from build123d import *

# Parameters (mm, degrees)
SKETCH1_R           = 1.96
BOSS_EXTRUDE1_DEPTH = 20
SKETCH2_R           = 3.45
BOSS_EXTRUDE2_DEPTH = 4
CUT_EXTRUDE1_DEPTH  = 2.7
FILLET1_R           = 0.2


with BuildPart() as part:
    # Sketch1 → Boss-Extrude1 (new body)
    with BuildSketch(Plane(origin=(0, 0, 0), x_dir=(1, 0, 0), z_dir=(0, 1, 0))):
        with Locations(Location((0, 0, 0), (0, 0, 270))):
            Circle(SKETCH1_R)
    extrude(amount=BOSS_EXTRUDE1_DEPTH)

    # Sketch2 → Boss-Extrude2 (add)
    with BuildSketch(Plane(origin=(0, 20, 0), x_dir=(1, 0, 0), z_dir=(0, 1, 0))):
        with Locations(Location((0, 0, 0), (0, 0, 270))):
            Circle(SKETCH2_R)
    extrude(amount=BOSS_EXTRUDE2_DEPTH)

    # Sketch3 → Cut-Extrude1 (cut)
    with BuildSketch(Plane(origin=(0, 24, 0), x_dir=(1, 0, 0), z_dir=(0, 1, 0))):
        Polygon((-0.053621876, 1.731220579), (-1.526091939, 0.819172383), (-1.472470063, -0.912048197), (0.053621876, -1.731220579), (1.526091939, -0.819172383), (1.472470063, 0.912048197), align=None)
    extrude(amount=-CUT_EXTRUDE1_DEPTH, mode=Mode.SUBTRACT)

    # Fillet1
    fillet1_edges = [part.edges().sort_by_distance(p)[0] for p in [
        (0, 20, -3.45),
        (0, 24, -3.45),
    ]]
    fillet(fillet1_edges, radius=FILLET1_R)


solid = part.part
Could you check a few things on this model? Use its own coordinates, in mm. A direction names the side the tool comes from. Round coordinates to 2 decimals unless told otherwise and drop trailing zeros. Write each loop counter-clockwise with the first axis right and the second up, starting at its lowest first coordinate (ties: lowest second). Pieces come first, ordered by that corner, then holes. Notation, with made-up numbers: (6.25, 1) -> (56.25, 1) arc R21 cw to (56.25, 20) -> close; hole circle Ø11 at (30, 69.25). An arc over 180 degrees is marked (long way). Use a Markdown table: item, result.
1. If we section it at A-A (y = 21.75): List the corners of the cut face in (x, z) for me, then the cut area to 3 significant figures.
Answer key:
| item | result |
|---|---|
| outline | circle Ø6.9 at (0, 0); hole (-1.53, -0.82) -> (-0.05, -1.73) -> (1.47, -0.91) -> (1.53, 0.82) -> (0.05, 1.73) -> (-1.47, 0.91) -> close |
| area | 29.6 mm^2 |
2. Which directions (+Z, -Z, +X, -X, +Y, -Y) give clear straight access to the entire face, cutting with the end or side of a thin tool? Please do faces 1 (the face through (0, 0, 0)), 2 (the face through (-0.78, 22.67, -1.28)), 3 (the face through (-2.12, 20, -0.05)).
Answer key:
| item | result |
|---|---|
| face 1 | +Z, -Z, +X, -X, -Y |
| face 2 | +Y |
| face 3 | -Y |
3. For pin 1 Ø1.5 at (y, z) = (8, 0.5) entering from +X; pin 2 Ø0.9 at (x, z) = (0.5, -0.5) entering from +Y; pin 3 Ø3 at (y, z) = (3.5, -2.5) entering from +X, each with a flat end and sliding along its axis, tell me the tip position at first contact or that it passes through.
Answer key:
| item | result |
|---|---|
| pin 1 | stops at x = 1.96 |
| pin 2 | stops at y = 21.3 |
| pin 3 | stops at x = 1.69 |
4. If we section it at B-B (z = 0): List the corners of the cut face in (x, y) for me.
Answer key:
| item | result |
|---|---|
| outline | (-3.45, 20.2) arc R0.2 ccw to (-3.25, 20) -> (-1.96, 20) -> (-1.96, 0) -> (1.96, 0) -> (1.96, 20) -> (3.25, 20) arc R0.2 ccw to (3.45, 20.2) -> (3.45, 23.8) arc R0.2 ccw to (3.25, 24) -> (1.5, 24) -> (1.5, 21.3) -> (-1.5, 21.3) -> (-1.5, 24) -> (-3.25, 24) arc R0.2 ccw to (-3.45, 23.8) -> close |
5. If we section it at C-C (y = 16): List the corners of the cut face in (x, z) for me.
Answer key:
| item | result |
|---|---|
| outline | circle Ø3.92 at (0, 0) |
6. We'd pull the mould along Z, two halves only. Please class faces 4 (the face through (0.72, 22.669, -1.316)), 5 (the face through (0.8, 24, -1.5)), 6 (the face through (2.332, 21.975, -2.543)): +Z half, -Z half, draft (parallel to the pull), parting line (faces both ways), or undercut.
Answer key:
| item | result |
|---|---|
| face 4 | undercut |
| face 5 | draft |
| face 6 | parting line |
7. Please list where these lines run through material, in increasing order: probe 1 along Y at (x, z) = (-0.5, 3.25); probe 2 along Z at (x, y) = (0.5, 22.25); probe 3 along X at (y, z) = (10.75, 0).
Answer key:
| item | result |
|---|---|
| probe 1 | y = 20 to 24 |
| probe 2 | z = -3.41 to -1.43, 1.45 to 3.41 |
| probe 3 | x = -1.96 to 1.96 |
